For this review, take the finished solid that the model builds, in its own axes (mm). Face numbers are marked on the shaded views. Coordinates: 2 decimals unless noted, no trailing zeros. Order: outer loops, then holes, each group sorted by start corner. A loop starts at its lowest first (then second) coordinate and runs counter-clockwise, first axis right, second up. Notation, with made-up numbers: (13, 26) -> (67, 26) arc R14 cw to (67, 51) -> close; hole circle Ø2 at (45, -17). An arc over 180 degrees is marked (long way). Write item = value, one per line. Start each with the question number.
1) Consider section D-D on y = -12.25. Give the boundary of the cut face in (x, z).
2) Insertion check: pin 1 Ø0.8 at (y, z) = (-12, 7.5) entering from -X; pin 2 Ø2 at (y, z) = (-10.5, 3) entering from +X; pin 3 Ø6 at (y, z) = (-11.5, 5.5) entering from +X. Each pin has a flat end and moves straight along its axis. Give the tip position at first contact, or say it passes through.
3) Consider section A-A on x = 0. Give the boundary of the cut face in (y, z), and give its area (3 significant figures).
4) Consider section B-B on z = 4.75. Give the boundary of the cut face in (x, y), and give its area (3 significant figures).
5) Draft analysis for pull direction X (two halves, no side actions). For the marked faces 1, 2 and 3, state which applies: +X half, -X half, draft (parallel to the pull), parting line (faces both ways), or undercut.
6) Wall thickness on probe 1 along Y at (x, z) = (0, 9.25); probe 2 along X at (y, z) = (-12.75, 15.25); probe 3 along X at (y, z) = (-13, 1.5): over which ranges is each line inside the solid? List them lowest first. Write a range as [from, to].
7) Consider section C-C on y = -19.75. Give the boundary of the cut face in (x, z), and give its area (3 significant figures).
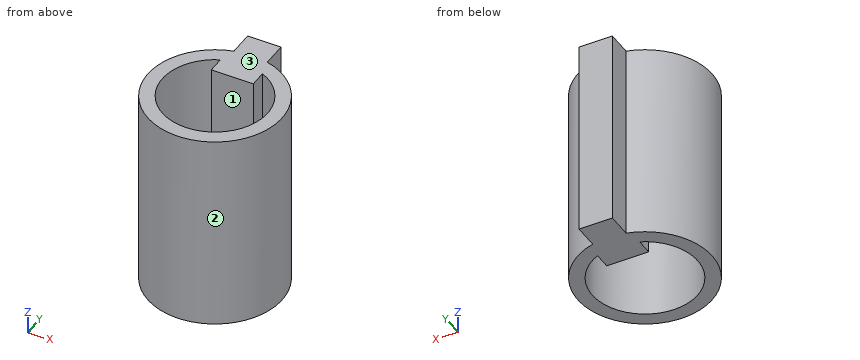
Autodesk Inventor part; units mm, degrees
ref_plane "YZ Plane" through (0, 0, 0) normal (1, 0, 0) x (0, 1, 0)
ref_plane "XZ Plane" through (0, 0, 0) normal (0, 1, 0) x (-1, 0, 0)
ref_plane "XY Plane" through (0, 0, 0) normal (0, 0, 1) x (1, 0, 0)
sketch "Sketch1" plane through (0, 0, 0) normal (0, 0, 1) x (1, 0, 0)
  arc A0 (-1.5875, -10.0999) -> (1.5875, -10.0999) centre (0, -16.2745) ccw
  line L0 (-1.5875, -10.0999) -> (-1.5875, -7.7187)
  line L1 (-1.5875, -7.7187) -> (1.5875, -7.7187)
  line L2 (1.5875, -7.7187) -> (1.5875, -10.0999)
  arc A1 (5.0716, -2.4388) -> (6.1971, -2.905) centre (6.228, -1.2388) ccw
  arc A2 (5.0716, -2.4388) -> (0.6091, -1.5512) centre (0, -16.2745) ccw
  arc A3 (-0.6091, -1.5512) -> (0.6091, -1.5512) centre (0, 0) ccw
  arc A4 (-0.6091, -1.5512) -> (-5.0716, -2.4388) centre (0, -16.2745) ccw
  arc A5 (-6.1971, -2.905) -> (-5.0716, -2.4388) centre (-6.228, -1.2388) ccw
  arc A6 (-6.1971, -2.905) -> (-9.9802, -5.4328) centre (0, -16.2745) ccw
  arc A7 (-10.8417, -6.2943) -> (-9.9802, -5.4328) centre (-11.5078, -4.7667) ccw
  arc A8 (-10.8417, -6.2943) -> (-13.3695, -10.0774) centre (0, -16.2745) ccw
  arc A9 (-13.8357, -11.2029) -> (-13.3695, -10.0774) centre (-15.0357, -10.0465) ccw
  arc A10 (-13.8357, -11.2029) -> (-14.7233, -15.6654) centre (0, -16.2745) ccw
  arc A11 (-14.7233, -16.8837) -> (-14.7233, -15.6654) centre (-16.2745, -16.2745) ccw
  arc A12 (-14.7233, -16.8837) -> (-13.8357, -21.3461) centre (0, -16.2745) ccw
  arc A13 (-13.3695, -22.4717) -> (-13.8357, -21.3461) centre (-15.0357, -22.5025) ccw
  arc A14 (-13.3695, -22.4717) -> (-10.8417, -26.2548) centre (0, -16.2745) ccw
  arc A15 (-9.9802, -27.1162) -> (-10.8417, -26.2548) centre (-11.5078, -27.7823) ccw
  arc A16 (-9.9802, -27.1162) -> (-6.1971, -29.644) centre (0, -16.2745) ccw
  arc A17 (-5.0716, -30.1102) -> (-6.1971, -29.644) centre (-6.228, -31.3102) ccw
  arc A18 (-5.0716, -30.1102) -> (-0.6091, -30.9978) centre (0, -16.2745) ccw
  arc A19 (0.6091, -30.9978) -> (-0.6091, -30.9978) centre (0, -32.549) ccw
  arc A20 (0.6091, -30.9978) -> (5.0716, -30.1102) centre (0, -16.2745) ccw
  arc A21 (6.1971, -29.644) -> (5.0716, -30.1102) centre (6.228, -31.3102) ccw
  arc A22 (6.1971, -29.644) -> (9.9802, -27.1162) centre (0, -16.2745) ccw
  arc A23 (10.8417, -26.2548) -> (9.9802, -27.1162) centre (11.5078, -27.7823) ccw
  arc A24 (10.8417, -26.2548) -> (13.3695, -22.4717) centre (0, -16.2745) ccw
  arc A25 (13.8357, -21.3461) -> (13.3695, -22.4717) centre (15.0357, -22.5025) ccw
  arc A26 (13.8357, -21.3461) -> (14.7233, -16.8837) centre (0, -16.2745) ccw
  arc A27 (14.7233, -15.6654) -> (14.7233, -16.8837) centre (16.2745, -16.2745) ccw
  arc A28 (14.7233, -15.6654) -> (13.8357, -11.2029) centre (0, -16.2745) ccw
  arc A29 (13.3695, -10.0774) -> (13.8357, -11.2029) centre (15.0357, -10.0465) ccw
  arc A30 (13.3695, -10.0774) -> (10.8417, -6.2943) centre (0, -16.2745) ccw
  arc A31 (9.9802, -5.4328) -> (10.8417, -6.2943) centre (11.5078, -4.7667) ccw
  arc A32 (9.9802, -5.4328) -> (6.1971, -2.905) centre (0, -16.2745) ccw
  line L3 (-2, -13.2745) -> (-2, -11.6919)
  arc A33 (-2, -11.6919) -> (2, -11.6919) centre (0, -16.2745) ccw
  line L4 (2, -13.2745) -> (2, -11.6919)
  line L5 (-2, -13.2745) -> (2, -13.2745)
extrude "Extrusion1" add sketch "Sketch1" along normal blind 19.05 contours L0 L1 L2 A0
properties part number "PG71 Adapter" material "Brass, Soft Yellow"
Answer sheet:
q1.outline = (-4.94, 0) -> (-2.97, 0) -> (-2.97, 19.05) -> (-4.94, 19.05) -> close; (-2, 0) -> (2, 0) -> (2, 19.05) -> (-2, 19.05) -> close; (2.97, 0) -> (4.94, 0) -> (4.94, 19.05) -> (2.97, 19.05) -> close
q2.pin_1 = -5.06
q2.pin_2 = 4.22
q2.pin_3 = 6.12
q3.outline = (-22.65, 0) -> (-21.27, 0) -> (-21.27, 19.05) -> (-22.65, 19.05) -> close; (-13.27, 0) -> (-7.72, 0) -> (-7.72, 19.05) -> (-13.27, 19.05) -> close
q3.area = 132 mm2
q4.outline = (-1.59, -10.1) arc R6.38 ccw (long way) to (1.59, -10.1) -> (1.59, -7.72) -> (-1.59, -7.72) -> close; hole (-2, -13.27) -> (-2, -11.69) arc R5 ccw (long way) to (2, -11.69) -> (2, -13.27) -> close
q4.area = 63.7 mm2
q5.face_1 = undercut
q5.face_2 = parting line
q5.face_3 = draft
q6.probe_1 = [-22.65, -21.27], [-13.27, -7.72]
q6.probe_2 = [-5.31, -3.55], [-2, 2], [3.55, 5.31]
q6.probe_3 = [-5.47, -3.78], [-2, 2], [3.78, 5.47]
q7.outline = (-5.34, 0) -> (-3.59, 0) -> (-3.59, 19.05) -> (-5.34, 19.05) -> close; (3.59, 0) -> (5.34, 0) -> (5.34, 19.05) -> (3.59, 19.05) -> close
q7.area = 66.7 mm2
